Autodesk Inventor part; units mm, degrees
ref_plane "YZ Plane" through (0, 0, 0) normal (1, 0, 0) x (0, 1, 0)
ref_plane "XZ Plane" through (0, 0, 0) normal (0, 1, 0) x (-1, 0, 0)
ref_plane "XY Plane" through (0, 0, 0) normal (0, 0, 1) x (1, 0, 0)
sketch "Sketch1" plane through (0, 0, 0) normal (0, 1, 0) x (-1, 0, 0)
  circle A0 centre (0, 0) radius 30
  dimension "d0" = 60
extrude "Extrusion1" add sketch "Sketch1" along normal blind 15.24
sketch "Sketch2" plane through (0, 15.24, 0) normal (0, 1, 0) x (1, 0, 0)
  circle A0 centre (0, 0) radius 8 construction
  circle A1 centre (-8, 0) radius 1.6
  circle A2 centre (0, -8) radius 1.6
  circle A3 centre (8, 0) radius 1.6
  circle A4 centre (0, 8) radius 1.6
  circle A5 centre (0, 0) radius 2.5 construction
  line L0 (-2.5, 1.4434) -> (0, 2.8868)
  line L1 (0, 2.8868) -> (2.5, 1.4434)
  line L2 (2.5, 1.4434) -> (2.5, -1.4434)
  line L3 (2.5, -1.4434) -> (0, -2.8868)
  line L4 (0, -2.8868) -> (-2.5, -1.4434)
  line L5 (-2.5, -1.4434) -> (-2.5, 1.4434)
  point P0 (-2.5, 0)
  dimension "d3" = 16
  dimension "d9" = 5
  dimension "d4" = 3.2
  dimension "d7" = 360
extrude "Extrusion2" cut sketch "Sketch2" against normal through all
properties part number "60mm_ThinWheel"
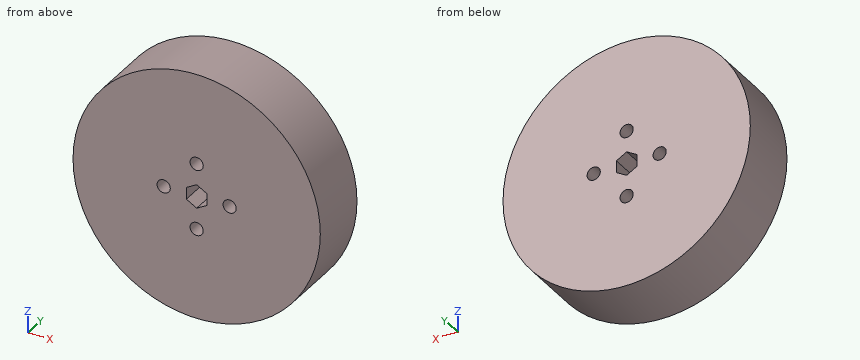
Verification items for the finished model (mm, model axes). Coordinates: 2 decimals unless noted, no trailing zeros. Loops run counter-clockwise (first coordinate to the right, second up) from the corner with the lowest first, then second, coordinate; pieces in that order, holes last. Notation, with made-up numbers: (51, -7.75) -> (98, -7.75) arc R20 cw to (98, 4.25) -> close; hole circle Ø10 at (51.5, 57.25). An arc over 180 degrees is marked (long way). Put each result on its own line as item: value.
1. Gauge pin test, flat ends, axial feed: P1, Ø5, axis at x = -3.5, y = 11.5, coming from the -Z side; P2, Ø1.5, axis at x = -9.5, y = 13, coming from the -Z side; P3, Ø5, axis at x = 10.5, y = 12, coming from the +Z side; P4, Ø3, axis at x = -8, z = 0, coming from the +Y side. Record the tip position at first contact, or that the pin passes through.
Result set:
P1: stops at z = -29.98
P2: stops at z = -28.7
P3: stops at z = 28.91
P4: passes through
2. Section check C-C, the plane z = 8. Record the boundary of the cut face in (x, y).
Result set:
outline: (-28.91, 0) -> (-1.6, 0) -> (-1.6, 15.24) -> (-28.91, 15.24) -> close; (1.6, 0) -> (28.91, 0) -> (28.91, 15.24) -> (1.6, 15.24) -> close
3. Section check B-B, the plane y = 13. Record the boundary of the cut face in (x, z), then the cut area to 3 significant figures.
Result set:
outline: circle Ø60 at (0, 0); hole circle Ø3.2 at (-8, 0); hole (-2.5, -1.44) -> (0, -2.89) -> (2.5, -1.44) -> (2.5, 1.44) -> (0, 2.89) -> (-2.5, 1.44) -> close; hole circle Ø3.2 at (0, -8); hole circle Ø3.2 at (0, 8); hole circle Ø3.2 at (8, 0)
area: 2,770 mm^2
4. Section check D-D, the plane x = 8. Record the boundary of the cut face in (y, z), then the cut area to 3 significant figures.
Result set:
outline: (0, -28.91) -> (15.24, -28.91) -> (15.24, -1.6) -> (0, -1.6) -> close; (0, 1.6) -> (15.24, 1.6) -> (15.24, 28.91) -> (0, 28.91) -> close
area: 833 mm^2
5. Thickness scan on line 1 (Z direction, x = 0, y = 4.25); line 2 (Z direction, x = 0.5, y = 12); line 3 (Z direction, x = -8, y = 6). Record the ranges inside material, lowest first.
Result set:
line 1: z = -30 to -9.6, -6.4 to -2.89, 2.89 to 6.4, 9.6 to 30
line 2: z = -30 to -9.52, -6.48 to -2.6, 2.6 to 6.48, 9.52 to 30
line 3: z = -28.91 to -1.6, 1.6 to 28.91
6. Section check A-A, the plane z = 0. Record the boundary of the cut face in (x, y).
Result set:
outline: (-30, 0) -> (-9.6, 0) -> (-9.6, 15.24) -> (-30, 15.24) -> close; (-6.4, 0) -> (-2.5, 0) -> (-2.5, 15.24) -> (-6.4, 15.24) -> close; (2.5, 0) -> (6.4, 0) -> (6.4, 15.24) -> (2.5, 15.24) -> close; (9.6, 0) -> (30, 0) -> (30, 15.24) -> (9.6, 15.24) -> close
